Can you work these out from the model? Positions are in its coordinate system, mm. Give positions to 0.01 mm unless a question says otherwise; leave off trailing zeros. Write each loop counter-clockwise with the first axis right and the second up, starting at its lowest first coordinate (ties: lowest second). Pieces come first, ordered by that corner, then holes. Notation, with made-up numbers: (51.5, 48) - (68.5, 48) arc R26 cw to (68.5, 62) - close; hole circle Ø2 at (-3, -32). An arc over 180 degrees is marked (long way). Return JSON: item names as keys, results as strings. Group by question number.
Autodesk Inventor part; units mm, degrees
ref_plane "YZ Plane" through (0, 0, 0) normal (1, 0, 0) x (0, 1, 0)
ref_plane "XZ Plane" through (0, 0, 0) normal (0, 1, 0) x (-1, 0, 0)
ref_plane "XY Plane" through (0, 0, 0) normal (0, 0, 1) x (1, 0, 0)
sketch "スケッチ1" plane through (0, 0, 0) normal (0, 0, 1) x (1, 0, 0)
  line L0 (17, 0) -> (17, 80)
  line L1 (17, 80) -> (0, 80)
  line L2 (0, 80) -> (0, 0) construction
  line L3 (-17, 0) -> (-17, 80)
  line L4 (-17, 80) -> (0, 80)
  line L5 (-17, 0) -> (17, 0)
  dimension "d75" = 34
  dimension "d86" = 80
extrude "プレート1" add sketch "スケッチ1" along normal blind 3
sketch "スケッチ3" plane through (0, 0, 3) normal (0, 0, 1) x (1, 0, 0)
  line L0 (-17, 80) -> (17, 80) construction
  line L1 (-17, 0) -> (-17, 80) construction
  line L2 (17, 80) -> (17, 0) construction
  line L3 (0, 0) -> (0, 80) construction
  line L4 (-17, 40) -> (17, 40) construction
  circle A0 centre (0, 60) radius 6
  circle A1 centre (0, 20) radius 6
  line L5 (17, 0) -> (-17, 0)
  point P0 (0, 0)
  dimension "d8" = 12
  dimension "d9" = 20
  dimension "d10" = 20
extrude "切り取り1" cut sketch "スケッチ3" against normal blind 3
sketch "スケッチ14" plane through (0, 0, 3) normal (0, 0, 1) x (1, 0, 0)
  line L0 (-17, 80) -> (17, 80)
  line L1 (-17, 0) -> (-17, 80)
  line L2 (17, 0) -> (-17, 0)
  line L3 (-37, 99.6299) -> (-37, -19.6299)
  line L4 (-37, -19.6299) -> (-17, -19.6299)
  line L5 (17, 0) -> (17, 80)
  line L6 (-17, -19.6299) -> (17, 0)
  line L7 (-37, 99.6299) -> (-17, 99.6299)
  line L8 (-17, 99.6299) -> (17, 80)
  line L9 (-27, 99.6299) -> (-27, -19.6299) construction
  line L10 (-27, 40) -> (-37, 40) construction
  circle A0 centre (-27, 89.6299) radius 2.25
  circle A1 centre (-27, -9.6299) radius 2.25
  circle A2 centre (-27, 40) radius 2.25
  point P0 (0, 0)
  dimension "d87" = 20
  dimension "d88" = 30
  dimension "d89" = 30
  dimension "d90" = 4.5
  dimension "d91" = 10
  dimension "d92" = 10
sheet face with bend "面3" sketch "スケッチ14" thickness 3 toward (0, 0, -1) bend radius 0 contours L1 L2 L6 L4 L3 L7 L8 L0
bend "曲げ5"
fillet "フィレット4" radius 10 6 edges at (-37, 99.6299, 1.5) (-17, 99.6299, 1.5) (17, 80, 1.5) (17, 0, 1.5) (-17, -19.6299, 1.5) (-37, -19.6299, 1.5)
equation "\"d11\" = Thickness"
equation "\"d89\" = d88"
equation "\"d92\" = d91"
equation "\"d5\" = Thickness"
equation "\"d10\" = d9"
equation "\"d94\" = BendReliefWidth"
equation "\"d96\" = MinimumRemnant"
equation "\"d95\" = BendReliefDepth"
equation "\"BendReliefWidth\" = Thickness"
equation "\"BendReliefDepth\" = 0.5 * Thickness"
equation "\"CornerReliefSize\" = 4 * Thickness"
equation "\"MinimumRemnant\" = 2 * Thickness"
equation "\"GapSize\" = Thickness"
properties part number "robocup_power_sw_plate" material "アルミニウム 6061"
1) Imagine slicing it at A-A, the plane y = 40. Write out the boundary of the cut face in (x, z).
2) Will this pin go through, and if not, where does the flat tip stop? pin 1 Ø3.5 at (x, y) = (-27, -9.63) entering from +Z.
3) I need wall thicknesses on line 1 along Y through (x, z) = (-2.5, 2.45); line 2 along Y through (x, z) = (0, 1.25); line 3 along X through (y, z) = (-8, 0.35). Which ranges of each line are inside material? Lowest first, please.
4) We'd pull the mould along Y, two halves only. Please class faces 1 (the face through (-37, 41, 2)), 2 (the face through (-24.854, -8.954, 1.521)), 3 (the face through (-1.53, -10.7, 1.52)): pulls with the +Y half, pulls with the -Y half, needs draft (parallel to the pull), parting line crosses it, or undercut.
5) Imagine slicing it at D-D, the plane y = 60. Write out the boundary of the cut face in (x, z), and give its area (3 significant figures).
6) Imagine slicing it at C-C, the plane x = 4. Write out the boundary of the cut face in (y, z), and give its area (3 significant figures).
7) Imagine slicing it at B-B, the plane z = 0.65. Write out the boundary of the cut face in (x, y), and give its area (3 significant figures).
Resolved:
{
 "1": {"outline": "(-37, 0) - (-29.25, 0) - (-29.25, 3) - (-37, 3) - close; (-24.75, 0) - (17, 0) - (17, 3) - (-24.75, 3) - close"},
 "2": {"pin 1": "through"},
 "3": {"line 1": "-11.26 to 14.55, 25.45 to 54.55, 65.45 to 91.26", "line 2": "-9.81 to 14, 26 to 54, 66 to 89.81", "line 3": "-37 to -28.55, -25.45 to 3.14"},
 "4": {"face 1": "needs draft", "face 2": "undercut", "face 3": "pulls with the -Y half"},
 "5": {"outline": "(-37, 0) - (-6, 0) - (-6, 3) - (-37, 3) - close; (6, 0) - (17, 0) - (17, 3) - (6, 3) - close", "area": "126 mm^2"},
 "6": {"outline": "(-7.51, 0) - (15.53, 0) - (15.53, 3) - (-7.51, 3) - close; (24.47, 0) - (55.53, 0) - (55.53, 3) - (24.47, 3) - close; (64.47, 0) - (87.51, 0) - (87.51, 3) - (64.47, 3) - close", "area": "231 mm^2"},
 "7": {"outline": "(-37, -9.63) arc R10 ccw to (-27, -19.63) - (-19.68, -19.63) arc R10 ccw to (-14.68, -18.29) - (12, -2.89) arc R10 ccw to (17, 5.77) - (17, 74.23) arc R10 ccw to (12, 82.89) - (-14.68, 98.29) arc R10 ccw to (-19.68, 99.63) - (-27, 99.63) arc R10 ccw to (-37, 89.63) - close; hole circle Ø4.5 at (-27, -9.63); hole circle Ø4.5 at (-27, 40); hole circle Ø4.5 at (-27, 89.63); hole circle Ø12 at (0, 20); hole circle Ø12 at (0, 60)", "area": "5,440 mm^2"}
}
